Design review of the part built by this model. Coordinates are the model's own, in mm. Face numbers are marked on the shaded views. A direction names the side the tool comes from. Give positions to 0.01 mm unless a question says otherwise; leave off trailing zeros. Write each loop counter-clockwise with the first axis right and the second up, starting at its lowest first coordinate (ties: lowest second). Pieces come first, ordered by that corner, then holes. Notation, with made-up numbers: M 80.5,14.5 L 108.5,14.5 A33 cw 108.5,50.5 Z; hole C -20,72 d7. An arc over 180 degrees is marked long. Use one line per item in the form item = value. Start each with the question number.
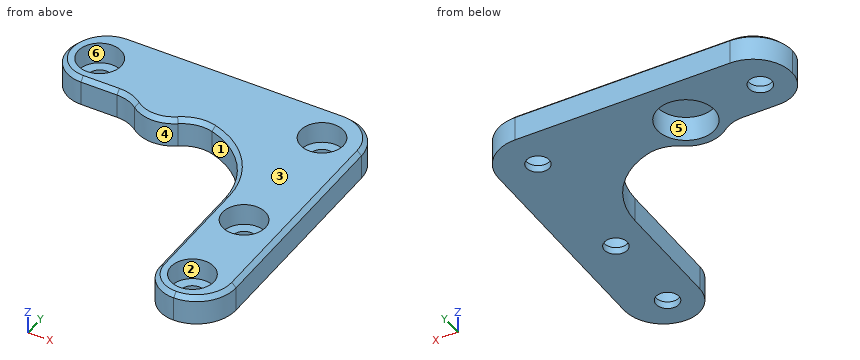
Solid Edge part; units mm, degrees
sketch "Sketch1" plane through (0, 0, 0) normal (0, 0, 1) x (1, 0, 0)
  line L0 (21, 15.5) -> (21, -14.5)
  arc A0 (15.5, -20) -> (21, -14.5) centre (15.5, -14.5) ccw
  arc A1 (11, -15.5) -> (15.5, -20) centre (15.5, -15.5) ccw
  line L1 (11, 0) -> (11, -15.5)
  arc A2 (-0.0878, 10.9996) -> (11, 0) centre (0, 0) cw
  arc A3 (-0.0878, 10.9996) -> (-8.4124, 11) centre (-4.25, 14) cw
  line L2 (-8.4124, 11) -> (-15.5, 11)
  arc A4 (-15.5, 11) -> (-20, 15.5) centre (-15.5, 15.5) cw
  arc A5 (-20, 15.5) -> (-14.5, 21) centre (-14.5, 15.5) cw
  line L3 (-14.5, 21) -> (15.5, 21)
  arc A6 (21, 15.5) -> (15.5, 21) centre (15.5, 15.5) ccw
extrude "Protrusion1" add sketch "Sketch1" along normal blind 4
fillet "Redondeo_1" radius 5 2 edges at (-0.0878, 10.9996, 2) (-8.4124, 11, 2)
sketch "Sketch2" plane through (0.5, 0.5, 0) normal (0, 0, -1) x (1, 0, 0)
  circle A0 centre (-4.75, -13.5) radius 4
extrude "VaciadoExtruido_1" cut sketch "Sketch2" against normal blind 3.5
hole "Agujero_1" at (-15.5, 15.5, 4) direction (0, 0, -1) diameter 3.2 end through all counterbore diameter 6 counterbore depth 3
hole "Hole1" at (15.5, 15.5, 4) direction (0, 0, -1) diameter 3.2 end through all counterbore diameter 6 counterbore depth 3
hole "Hole2" at (15.5, -3.15, 4) direction (0, 0, -1) diameter 3.2 end through all counterbore diameter 6 counterbore depth 3
hole "Hole3" at (15.5, -15.5, 4) direction (0, 0, -1) diameter 3.2 end through all counterbore diameter 6 counterbore depth 3
chamfer "Chaflán_1" distance 0.6 angle 45 13 edges at (0.5, 21, 4) (19.3891, 19.3891, 4) (21, 0.5, 4) (19.3891, -18.3891, 4) (12.318, -18.682, 4) (11, -7.75, 4) (8.7852, 6.6197, 4) (0.8013, 10.6942, 4) (-4.3484, 8.8701, 4) (-8.8442, 10.7298, 4) (-12.9828, 11, 4) (-18.682, 12.318, 4) (-18.3891, 19.3891, 4)
1. To check wall thickness, follow L1, parallel to X at y = 15.5, z = 0.45; L2, parallel to Y at x = 2, z = 2.4; L3, parallel to X at y = -18, z = 3.05. State the ranges of each line that lie inside material, in increasing order.
2. For the marked faces 4, 5 and 6, list the 3-axis set-ups (+Z, -Z, +X, -X, +Y, -Y) from which the entire face can be reached by the end or side of a thin tool; tool diameter is ignored.
3. Draft analysis for pull direction Y (two halves, no side actions). For the marked faces 1, 2 and 3, state which applies: pulls with the +Y half, pulls with the -Y half, needs draft (parallel to the pull), parting line crosses it, or undercut.
4. We need section B-B (x = -4.25). State the section outline as (y, z) points.
5. Clearance check with flat-ended pins moving along their axes: pin 1 Ø7 at (x, y) = (15.5, 15.5) entering from -Z; pin 2 Ø5 at (x, y) = (15.5, -3.15) entering from +Z; pin 3 Ø4 at (x, y) = (-5, 15.5) entering from -Z. State where each tip first meets the part, or that it passes through.
6. We need section A-A (z = 2.2). Give the number of separate pieces and of enclosed holes in the cut face, and give its area (3 significant figures).
Answer block:
q1.L1 = -20 to -17.1, -13.9 to -7.96, -0.54 to 13.9, 17.1 to 21
q1.L2 = 10.76 to 21
q1.L3 = 11.76 to 13.84, 17.16 to 19.74
q2.face_4 = +Z, -Z, -Y
q2.face_5 = -Z
q2.face_6 = +Z
q3.face_1 = pulls with the -Y half
q3.face_2 = undercut
q3.face_3 = needs draft
q4.outline = M 8.87,0 L 10,0 L 10,3.5 L 18,3.5 L 18,0 L 21,0 L 21,3.4 L 20.4,4 L 9.47,4 L 8.87,3.4 Z
q5.pin_1 = 0
q5.pin_2 = 1
q5.pin_3 = 3.5
q6.separate_pieces = 1
q6.enclosed_holes = 5
q6.area = 568 mm^2
